Build history of the part. All positions in model axes, mm. A direction names the side the tool comes from. Round coordinates to 2 decimals unless told otherwise and drop trailing zeros. Loops run counter-clockwise (first coordinate to the right, second up) from the corner with the lowest first, then second, coordinate; pieces in that order, holes last. Notation, with made-up numbers: M 66,-34.75 L 102,-34.75 A17 ccw 102,-9.75 Z; hole C 64.5,24.25 d9. An arc over 180 degrees is marked long. One line per item, written item: value.
```python
from build123d import *

# Parameters (mm, degrees)
BOSS_EXTRU_1_DEPTH      = 13
ESQUISSE2_R             = 2.5
ENL_V_MAT_EXTRU_1_DEPTH = 77.583287994


with BuildPart() as part:
    # Esquisse1 → Boss.-Extru.1 (new body)
    with BuildSketch(Plane.XY):
        Polygon((0, 0), (0, 40), (64, 40), (64, 0), (60, 0), (60, 36), (4, 36), (4, 0), align=None)
    extrude(amount=BOSS_EXTRU_1_DEPTH)

    # Esquisse2 → Enlèv. mat.-Extru.1 (cut, through all)
    with BuildSketch(Plane(origin=(64, 0, 0), x_dir=(0, 0, -1), z_dir=(1, 0, 0))):
        with Locations((-6.5, 10)):
            Circle(ESQUISSE2_R)
    extrude(amount=-ENL_V_MAT_EXTRU_1_DEPTH, mode=Mode.SUBTRACT)


solid = part.part
```
Item 1: Slice it at B-B, the plane z = 6.5. Give the cut face in (x, y), and give its area (3 significant figures).
Check values:
outline: M 0,0 L 4,0 L 4,7.5 L 0,7.5 Z; M 0,12.5 L 4,12.5 L 4,36 L 60,36 L 60,12.5 L 64,12.5 L 64,40 L 0,40 Z; M 60,0 L 64,0 L 64,7.5 L 60,7.5 Z
area: 504 mm2
Item 2: Slice it at D-D, the plane z = 12. Give the cut face in (x, y), and give its area (3 significant figures).
Check values:
outline: M 0,0 L 4,0 L 4,36 L 60,36 L 60,0 L 64,0 L 64,40 L 0,40 Z
area: 544 mm2
Item 3: Pull direction X, two halves, no side cores. Call faces 1 (the face through (2, 8, 5)), 2 (the face through (32, 36, 6)), 3 (the face through (64, 20, 6)): pulls with the +X half, pulls with the -X half, needs draft (parallel to the pull), parting line crosses it, or undercut.
Check values:
face 1: needs draft
face 2: undercut
face 3: pulls with the +X half
Item 4: Slice it at A-A, the plane y = 30. Give the cut face in (x, z).
Check values:
outline: M 0,0 L 4,0 L 4,13 L 0,13 Z; M 60,0 L 64,0 L 64,13 L 60,13 Z
Item 5: Slice it at C-C, the plane y = 10. Give the cut face in (x, z), and give its area (3 significant figures).
Check values:
outline: M 0,0 L 4,0 L 4,4 L 0,4 Z; M 0,9 L 4,9 L 4,13 L 0,13 Z; M 60,0 L 64,0 L 64,4 L 60,4 Z; M 60,9 L 64,9 L 64,13 L 60,13 Z
area: 64.0 mm2
Item 6: Which spindle directions (+Z, -Z, +X, -X, +Y, -Y) get a long thin tool onto all of the face, cutting with end or side? Do faces 4 (the face through (60, 18, 6)), 5 (the face through (62, 0, 6)). Say none if no direction does.
Check values:
face 4: +Z, -Z, -Y
face 5: +Z, -Z, +X, -X, -Y
Item 7: Wall check: line 1 along X through (y, z) = (28.5, 4.75); line 2 along Y through (x, z) = (2.15, 6.5); line 3 along Y through (x, z) = (24, 12.25). Give the ranges that are in metal, low to high.
Check values:
line 1: x = 0 to 4, 60 to 64
line 2: y = 0 to 7.5, 12.5 to 40
line 3: y = 36 to 40
Item 8: Drop a flat-ended pin along its axis: P1, Ø1.5, axis at x = 54, z = 5, coming from the -Y side. Give the stop position or say it passes through.
Check values:
P1: stops at y = 36
